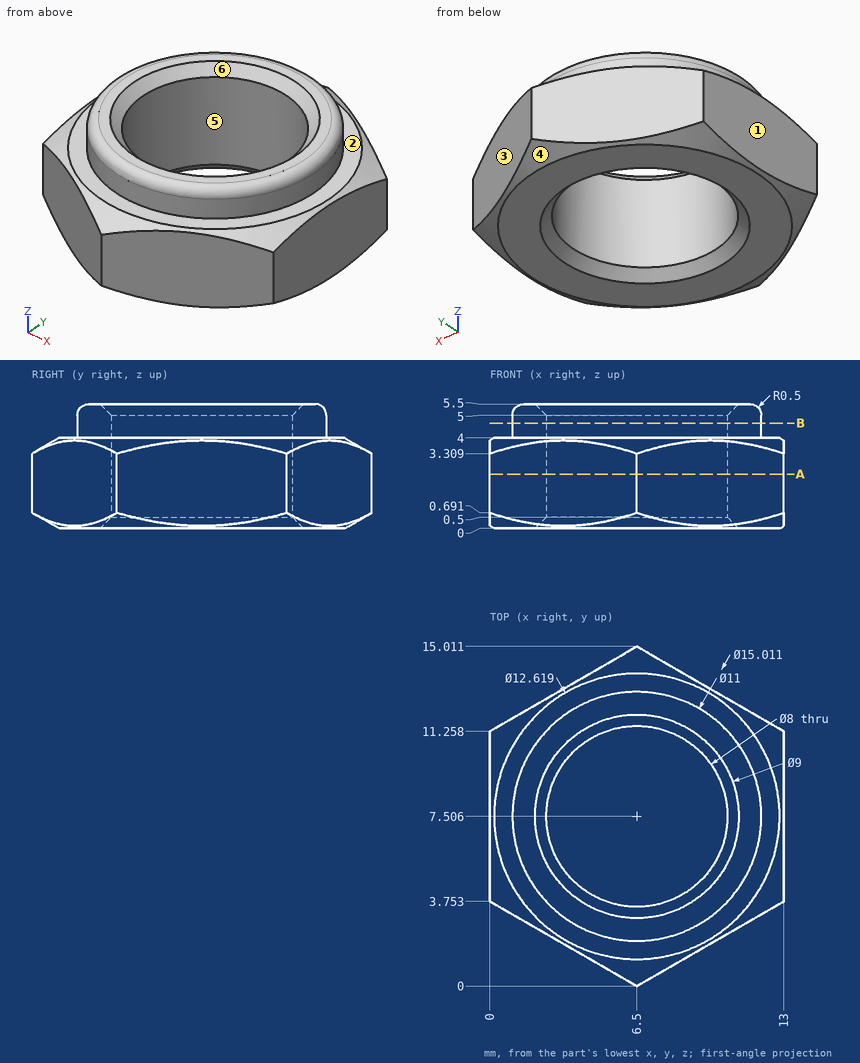
Source: three-view drawing plus pictorial views. Frame: mm from the lowest corner of the part. A direction names the side the tool comes from. Coordinates: 2 decimals unless noted, no trailing zeros. Order: outer loops, then holes, each group sorted by start corner. A loop starts at its lowest first (then second) coordinate and runs counter-clockwise, first axis right, second up. Notation, with made-up numbers: M 13.5,57 L 49.5,57 A25 ccw 49.5,77 Z; hole C 61.25,63.5 d10. An arc over 180 degrees is marked long. One line per question, with ' | ' between items. Start each with the question number.
Item 1: Cut plane B-B, the plane z = 4.65. Return the cut outline in (x, y) (1 decimal).
Item 2: Ray query, probe 1 along Z at (x, y) = (10, 3); probe 2 along X at (y, z) = (9.25, 3.2); probe 3 along X at (y, z) = (10.5, 5.35) (1 decimal). Return the intervals inside material, ascending. Write a range as [from, to].
Item 3: Cut plane A-A, the plane z = 2.4. Return the cut outline in (x, y) (1 decimal).
Item 4: Draft query along X for the marked faces 3, 4, 5 and 6. Return one class per face: released by +X, released by -X, zero draft, split by the parting line, or undercut.
Item 5: Pin query (flat end, axial travel): pin 1 Ø1 at (x, z) = (4.5, 3.5) entering from -Y (1 decimal); pin 2 Ø1.5 at (x, y) = (6, 4) entering from -Z. Return the tip coordinate at first contact, or that it passes through.
Item 6: Set-up query: the marked faces 1 and 2. Return all of +Z, -Z, +X, -X, +Y, -Y with unobstructed straight access to the full face (end or side cutting, diameter ignored); none if empty.
A:
1) outline: C 6.5,7.5 d11; hole C 6.5,7.5 d8
2) probe 1: z = [0, 4] | probe 2: x = [0, 2.9], [10.1, 13] | probe 3: x = [2.1, 3.3], [9.7, 10.9]
3) outline: M 0,3.8 L 6.5,0 L 13,3.8 L 13,11.3 L 6.5,15 L 0,11.3 Z; hole C 6.5,7.5 d8
4) face 3: released by +X | face 4: split by the parting line | face 5: undercut | face 6: undercut
5) pin 1: stops at y = 0.9 | pin 2: stops at z = 0.21
6) face 1: +Z, -Z, -X, +Y, -Y | face 2: +Z
